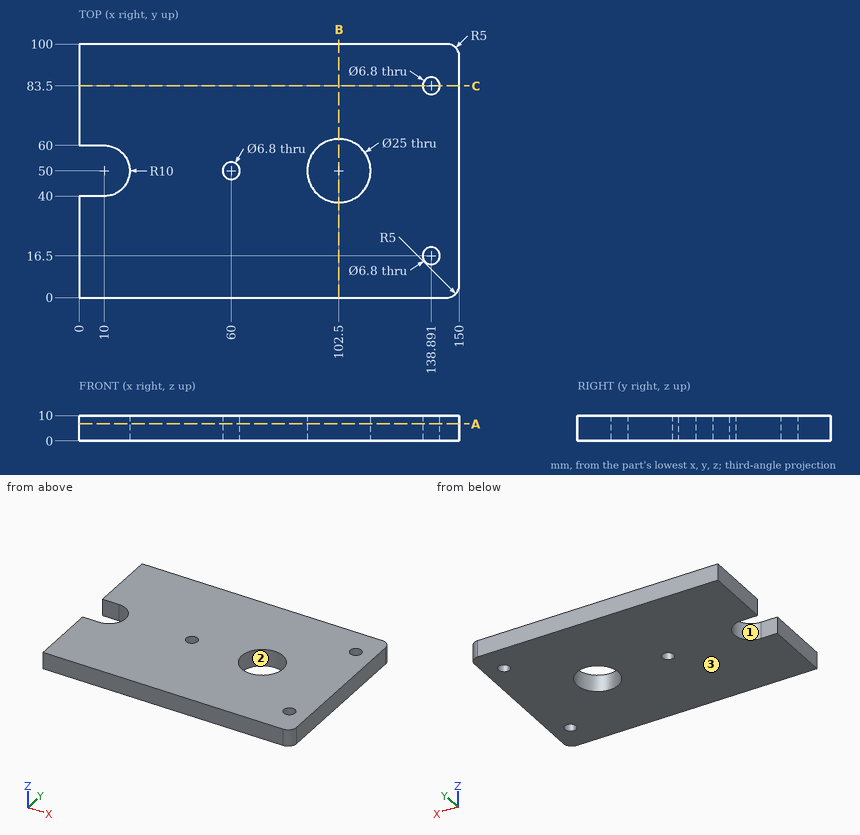
Answer from the drawing. Dimensions are ordinates in mm from the lowest x, y and z of the part. Round coordinates to 2 decimals unless told otherwise and drop trailing zeros. Write each loop counter-clockwise with the first axis right and the second up, starting at its lowest first coordinate (ties: lowest second). Pieces come first, ordered by that corner, then holes. Notation, with made-up numbers: (46, -27) -> (67, -27) arc R25 cw to (67, 5) -> close; hole circle Ø7 at (29.25, 59). An arc over 180 degrees is marked (long way). Answer in a Markdown table with one row per item. Add a question column.
1) Find section A-A, the plane z = 6.75. Determine the outline of the cut face in (x, y), and give its area (3 significant figures).
2) Consider line 1 (X direction, y = 48, z = 9.25); line 2 (Y direction, x = 60, z = 5.5); line 3 (X direction, y = 18.5, z = 2.75). Determine where each line is inside the solid, lowest interval first.
3) Given P1, Ø11, axis at x = 138.891, y = 83.5, coming from the -Z side, flat-ended and moving along its own axis, determine where the tip first touches the part or whether it passes through.
4) Find section B-B, the plane x = 102.5. Determine the outline of the cut face in (y, z).
5) Find section C-C, the plane y = 83.5. Determine the outline of the cut face in (x, z), and give its area (3 significant figures).
6) Determine the mould class of the marked faces 1, 2 and 3 for opening direction X: pulls with the +X half, pulls with the -X half, needs draft (parallel to the pull), parting line crosses it, or undercut.
Findings below:
| question | item | result |
|---|---|---|
| 1 | outline | (0, 0) -> (145, 0) arc R5 ccw to (150, 5) -> (150, 95) arc R5 ccw to (145, 100) -> (0, 100) -> (0, 60) -> (10, 60) arc R10 cw to (10, 40) -> (0, 40) -> close; hole circle Ø6.8 at (60, 50); hole circle Ø25 at (102.5, 50); hole circle Ø6.8 at (138.89, 16.5); hole circle Ø6.8 at (138.89, 83.5) |
| 1 | area | 14,000 mm² |
| 2 | line 1 | 19.8 to 57.25, 62.75 to 90.16, 114.84 to 150 |
| 2 | line 2 | 0 to 46.6, 53.4 to 100 |
| 2 | line 3 | 0 to 136.14, 141.64 to 150 |
| 3 | P1 | z = 0 |
| 4 | outline | (0, 0) -> (37.5, 0) -> (37.5, 10) -> (0, 10) -> close; (62.5, 0) -> (100, 0) -> (100, 10) -> (62.5, 10) -> close |
| 5 | outline | (0, 0) -> (135.49, 0) -> (135.49, 10) -> (0, 10) -> close; (142.29, 0) -> (150, 0) -> (150, 10) -> (142.29, 10) -> close |
| 5 | area | 1,430 mm² |
| 6 | face 1 | pulls with the -X half |
| 6 | face 2 | undercut |
| 6 | face 3 | needs draft |
